from build123d import *

# Parameters (mm, degrees)
SKETCH1_R           = 0.5
BOSS_EXTRUDE1_DEPTH = 0.762
FILLET1_R           = 2.54
FILLET2_R           = 0.507185


with BuildPart() as part:
    # Sketch1 → Boss-Extrude1 (new body)
    with BuildSketch(Plane.XY):
        with BuildLine():
            Line((-0.3175, 18.2372), (0.3175, 18.2372))
            Line((0.3175, 18.2372), (1.1811, 16.4592))
            Line((1.1811, 16.4592), (1.1811, 2.947138916))
            ThreePointArc((1.1811, 2.947138916), (0, -3.175), (-1.1811, 2.947138916))
            Line((-1.1811, 2.947138916), (-1.1811, 16.4592))
            Line((-1.1811, 16.4592), (-0.3175, 18.2372))
        make_face()
        Circle(SKETCH1_R, mode=Mode.SUBTRACT)
    extrude(amount=BOSS_EXTRUDE1_DEPTH)

    # Fillet1
    fillet1_edges = [part.edges().sort_by_distance(p)[0] for p in [
        (1.1811, 16.4592, 0.381),
        (1.1811, 2.947138916, 0.381),
        (-1.1811, 2.947138916, 0.381),
        (-1.1811, 16.4592, 0.381),
    ]]
    fillet(fillet1_edges, radius=FILLET1_R)

    # Fillet2
    fillet2_edges = [part.edges().sort_by_distance(p)[0] for p in [
        (-0.3175, 18.2372, 0.381),
        (0.3175, 18.2372, 0.381),
    ]]
    fillet(fillet2_edges, radius=FILLET2_R - 0.0001)  # a hair under: the kernel refuses the full size


solid = part.part
Check sheet for the modelled part. Datum: model origin and axes. Units: mm. Give positions to 0.01 mm unless a question says otherwise; leave off trailing zeros. Write each loop counter-clockwise with the first axis right and the second up, starting at its lowest first coordinate (ties: lowest second). Pieces come first, ordered by that corner, then holes. Notation, with made-up numbers: (38.5, -25) -> (61.5, -25) arc R14 cw to (61.5, 1) -> close; hole circle Ø5 at (45, 83.5). An arc over 180 degrees is marked (long way). One line per item, written item: value. Start each with the question number.
Item 1: Draft check along Y on faces 1 (the cylindrical face through (0.108, -3.173, 0.376)), 2 (the flat face through (0, 5, 0)), 3 (the cylindrical face through (-1.407, 3.291, 0.386)), 4 (the cylindrical face through (-0.108, -0.488, 0.376)). Enter one of: +Y half, -Y half, draft (parallel to the pull), parting line (faces both ways), or undercut.
Item 2: Section check A-A on y = -0.25. Record the cut outline in (x, z).
Item 3: Section check D-D on y = 12.75. Record the cut outline in (x, z).
Item 4: Material ranges on probe 1 along Y at (x, z) = (0, 0.4) (3 decimals); probe 2 along X at (y, z) = (10.25, 0.7); probe 3 along Y at (x, z) = (1.5, 0.1), recorded low to high. Write a range as from..to.
Item 5: Section check C-C on x = 0.25. Record the cut outline in (y, z), then the cut area to 3 significant figures.
Results list:
1. face 1: parting line
1. face 2: draft
1. face 3: +Y half
1. face 4: undercut
2. outline: (-3.17, 0) -> (-0.43, 0) -> (-0.43, 0.76) -> (-3.17, 0.76) -> close; (0.43, 0) -> (3.17, 0) -> (3.17, 0.76) -> (0.43, 0.76) -> close
3. outline: (-1.18, 0) -> (1.18, 0) -> (1.18, 0.76) -> (-1.18, 0.76) -> close
4. probe 1: -3.175..-0.5, 0.5..18.237
4. probe 2: -1.18..1.18
4. probe 3: -2.8..3.11
5. outline: (-3.17, 0) -> (-0.43, 0) -> (-0.43, 0.76) -> (-3.17, 0.76) -> close; (0.43, 0) -> (18.17, 0) -> (18.17, 0.76) -> (0.43, 0.76) -> close
5. area: 15.6 mm²
